```python
from build123d import *

# Parameters (mm, degrees)
F1_DEPTH = 100
F2_W     = 10
F2_H     = 70
F3_DEPTH = 70
F5_DEPTH = 10
F6_R     = 4.25
F7_DEPTH = 10
F8_R     = 4.25
F9_DEPTH = 10
F10_R    = 2


with BuildPart() as f1:
    # F0 (on Right) → F1 (new body, symmetric)
    with BuildSketch(Plane.YZ):
        Polygon((5, -118.2), (5, 81.8), (-5, 81.8), (-5, 5), (-110.4780795566, 5), (-110.4780795566, -5), (-5, -5), (-5, -118.2), align=None)
    extrude(amount=F1_DEPTH, both=True)

    # F2 (on face) → F3 (join)
    with BuildSketch(Plane.XZ.offset(5)):
        with Locations((0, -40)):
            Rectangle(F2_W, F2_H)
    extrude(amount=F3_DEPTH)

    # F4 (on face) → F5 (cut)
    with BuildSketch(Plane(origin=(-5, 0, 0), x_dir=(0, -1, 0), z_dir=(-1, 0, 0))):
        Polygon((75, -75), (75, -5), (5, -75), align=None)
    extrude(amount=-F5_DEPTH, mode=Mode.SUBTRACT)

    # F6 (on face) → F7 (cut)
    with BuildSketch(Plane.XZ.offset(5)):
        with Locations((85, -103.2)):
            Circle(F6_R)
        with Locations((-85, -103.2)):
            Circle(F6_R)
    extrude(amount=-F7_DEPTH, mode=Mode.SUBTRACT)

    # F8 (on face) → F9 (cut)
    with BuildSketch(Plane.XZ.offset(5)):
        with Locations((-85, 66.8)):
            Circle(F8_R)
        with Locations((85, 66.8)):
            Circle(F8_R)
    extrude(amount=-F9_DEPTH, mode=Mode.SUBTRACT)

    # F10
    f10_edges = [f1.edges().sort_by_distance(p)[0] for p in [
        (-52.5, -5, -5),
        (52.5, -5, -5),
        (-5, -40, -5),
        (-5, -5, -40),
        (5, -5, -40),
        (5, -40, -5),
        (0, -5, 5),
    ]]
    fillet(f10_edges, radius=F10_R)


solid = f1.part
```
The model under review builds one solid part; all positions refer to its coordinate system, in mm. A direction names the side the tool comes from. Give positions to 0.01 mm unless a question says otherwise; leave off trailing zeros. Write each loop counter-clockwise with the first axis right and the second up, starting at its lowest first coordinate (ties: lowest second). Pieces come first, ordered by that corner, then holes.
(1) For P1, Ø6, axis at y = -28, z = -43.5, coming from the -X side; P2, Ø4, axis at y = -21.5, z = -49, coming from the +X side; P3, Ø2, axis at y = -33, z = -50.5, coming from the -X side; P4, Ø22.5, axis at x = -44, z = 31.5, coming from the -Y side, all flat-tipped, find the tip position at first contact; note any pin that passes through.
(2) Consider section D-D, the plane z = -26.5. Give the boundary of the cut face in (x, y), and give its area (3 significant figures).
(3) The part is to be moulded in two halves that separate along Z. For faces 1 (the cylindrical face through (80.754, -0.07, -103.013)), 2 (the flat face through (-5, -25, -26)), 3 (the cylindrical face through (-89.246, -0.07, -103.013)), 4 (the flat face through (0, -40, -40)), say which applies: released by +Z, released by -Z, zero draft, split by the parting line, or undercut.
(4) Consider section B-B, the plane x = -85. Give the boundary of the cut face in (y, z), and give its area (3 significant figures).
(5) Tool access review of faces 5 (the flat face through (5, -25, -26)), 6 (the flat face through (1, -5, 45)), 7 (the flat face through (24, -5, -62)): name each direction out of +Z, -Z, +X, -X, +Y, -Y from which nothing blocks a thin tool from reaching the whole face with its end or side.
(6) To check wall thickness, follow L1, parallel to Z at x = -85, y = -2.75; L2, parallel to X at y = 0, z = -103; L3, parallel to Y at x = 83, z = -20. State the ranges of each line that lie inside material, in increasing order.
(7) Consider section A-A, the plane z = -103.2. Give the boundary of the cut face in (x, y).
(8) Consider section C-C, the plane x = -2. Give the boundary of the cut face in (y, z).
Returned:
1. P1: stops at x = -5
1. P2: stops at x = 5
1. P3: passes through
1. P4: stops at y = -5
2. outline: (-100, -5) - (-7, -5) arc R2 cw to (-5, -7) - (-5, -53.5) - (5, -53.5) - (5, -7) arc R2 cw to (7, -5) - (100, -5) - (100, 5) - (-100, 5) - close
2. area: 2,490 mm2
3. face 1: undercut
3. face 2: zero draft
3. face 3: undercut
3. face 4: released by -Z
4. outline: (-110.48, -5) - (-7, -5) arc R2 cw to (-5, -7) - (-5, -98.95) - (5, -98.95) - (5, 62.55) - (-5, 62.55) - (-5, 7) arc R2 cw to (-7, 5) - (-110.48, 5) - close; (-5, -118.2) - (5, -118.2) - (5, -107.45) - (-5, -107.45) - close; (-5, 71.05) - (5, 71.05) - (5, 81.8) - (-5, 81.8) - close
4. area: 2,890 mm2
5. face 5: -Z, +X, -Y
5. face 6: +Z, +X, -X, -Y
5. face 7: -Z, -Y
6. L1: z = -118.2 to -107.45, -98.95 to 62.55, 71.05 to 81.8
6. L2: x = -100 to -89.25, -80.75 to 80.75, 89.25 to 100
6. L3: y = -5 to 5
7. outline: (-100, -5) - (-89.25, -5) - (-89.25, 5) - (-100, 5) - close; (-80.75, -5) - (80.75, -5) - (80.75, 5) - (-80.75, 5) - close; (89.25, -5) - (100, -5) - (100, 5) - (89.25, 5) - close
8. outline: (-110.48, -5) - (-75, -5) - (-5, -75) - (-5, -118.2) - (5, -118.2) - (5, 81.8) - (-5, 81.8) - (-5, 7) arc R2 cw to (-7, 5) - (-110.48, 5) - close
